from build123d import *

# Parameters (mm, degrees)
SKETCH1_R           = 10
BOSS_EXTRUDE1_DEPTH = 24


with BuildPart() as part:
    # Sketch1 → Boss-Extrude1 (new body)
    with BuildSketch(Plane.XY):
        with BuildLine():
            Line((24.140215409, 6.5), (11.587303396, 53.12))
            ThreePointArc((11.587303396, 53.12), (0, 62), (-11.587303396, 53.12))
            Line((-11.587303396, 53.12), (-24.140215409, 6.5))
            ThreePointArc((-24.140215409, 6.5), (-24.936514863, 1.780512988), (-24.81883517, -3.004233816))
            ThreePointArc((-24.81883517, -3.004233816), (-30.762049538, -19.776348187), (-47.717387131, -25.174694658))
            ThreePointArc((-47.717387131, -25.174694658), (-61.385060233, -49.766289136), (-35, -40))
            ThreePointArc((-35, -40), (-25.668051324, -25.370335536), (-8.412024081, -23.542256707))
            ThreePointArc((-8.412024081, -23.542256707), (0, -25), (8.412024081, -23.542256707))
            ThreePointArc((8.412024081, -23.542256707), (25.668051324, -25.370335536), (35, -40))
            ThreePointArc((35, -40), (61.385060233, -49.766289136), (47.717387131, -25.174694658))
            ThreePointArc((47.717387131, -25.174694658), (30.762049538, -19.776348187), (24.81883517, -3.004233816))
            ThreePointArc((24.81883517, -3.004233816), (24.936514863, 1.780512988), (24.140215409, 6.5))
        make_face()
        with Locations((50, -40)):
            Circle(SKETCH1_R, mode=Mode.SUBTRACT)
        with Locations(Location((-50, -40, 0), (0, 0, 180))):
            Circle(SKETCH1_R, mode=Mode.SUBTRACT)
        with BuildLine():
            Line((4.769696007, 51.5), (19.078784028, 6))
            ThreePointArc((19.078784028, 6), (0, -20), (-19.078784028, 6))
            Line((-19.078784028, 6), (-4.769696007, 51.5))
            ThreePointArc((-4.769696007, 51.5), (0, 55), (4.769696007, 51.5))
        make_face(mode=Mode.SUBTRACT)
    extrude(amount=BOSS_EXTRUDE1_DEPTH)


solid = part.part
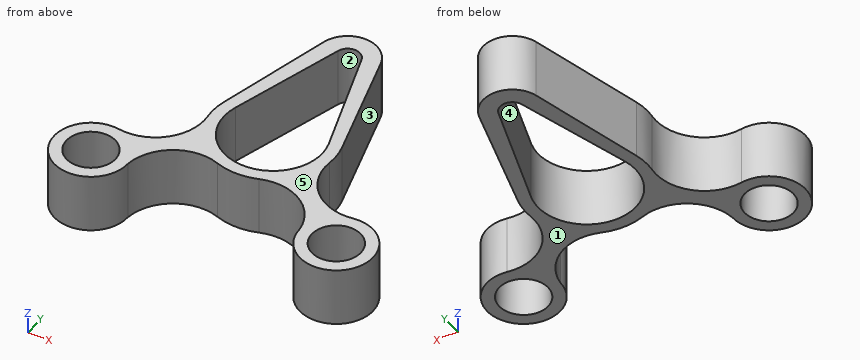
Can you work these out from the model? Positions are in its coordinate system, mm. Face numbers are marked on the shaded views. A direction names the side the tool comes from. Round coordinates to 2 decimals unless told otherwise and drop trailing zeros. Write each loop counter-clockwise with the first axis right and the second up, starting at its lowest first coordinate (ties: lowest second). Pieces come first, ordered by that corner, then holes. Notation, with made-up numbers: (-38, 10.25) -> (21, 10.25) arc R18 ccw to (21, 18.25) -> close; hole circle Ø10 at (-23.75, -3). An arc over 180 degrees is marked (long way). One line per question, with ' | ' between items. Start each with the question number.
1) I'm going to push flat-ended pins straight in: P1, Ø12, axis at y = 19.5, z = 20.5, coming from the +X side; P2, Ø1, axis at y = 25.5, z = 19, coming from the -X side; P3, Ø10, axis at x = 10, y = 46.5, coming from the -Z side; P4, Ø12, axis at x = -50, y = -40, coming from the -Z side. Where does each tip first touch, or does it pass through?
2) Suppose I cut it at A-A on y = 0. Write out the boundary of the cut face in (x, z), then the cut area to 3 significant figures.
3) Suppose I cut it at C-C on z = 19.75. Write out the boundary of the cut face in (x, y), then the cut area to 3 significant figures.
4) I need wall thicknesses on line 1 (Y direction, x = 0, z = 8.75); line 2 (Y direction, x = -50, z = 7.75); line 3 (X direction, y = 0, z = 7). Which ranges of each line are inside material? Lowest first, please. Write a range as [from, to].
5) If we mould it in two halves opening along Y, with no side actions, what happens to the marked faces 1, 2 and 3? For each: released by +Y, released by -Y, zero draft, split by the parting line, or undercut.
6) On a 3-axis mill with a long thin cutter (end or side, diameter ignored), from which of +Z, -Z, +X, -X, +Y, -Y can I reach the whole of each face in a straight line? I mean the marked faces 4 and 5. Say none if no direction works.
7) Suppose I cut it at B-B on x = -50. Write out the boundary of the cut face in (y, z).
Return value:
1) P1: stops at x = 22.26 | P2: stops at x = -19.16 | P3: stops at z = 0 | P4: passes through
2) outline: (-25, 0) -> (-20, 0) -> (-20, 24) -> (-25, 24) -> close; (20, 0) -> (25, 0) -> (25, 24) -> (20, 24) -> close | area: 240 mm2
3) outline: (-47.72, -25.17) arc R15 ccw (long way) to (-35, -40) arc R20 cw to (-8.41, -23.54) arc R25 ccw to (8.41, -23.54) arc R20 cw to (35, -40) arc R15 ccw (long way) to (47.72, -25.17) arc R20 cw to (24.82, -3) arc R25 ccw to (24.14, 6.5) -> (11.59, 53.12) arc R12 ccw to (-11.59, 53.12) -> (-24.14, 6.5) arc R25 ccw to (-24.82, -3) arc R20 cw to start; hole circle Ø20 at (-50, -40); hole (-19.08, 6) arc R20 ccw (long way) to (19.08, 6) -> (4.77, 51.5) arc R5 ccw to (-4.77, 51.5) -> close; hole circle Ø20 at (50, -40) | area: 2,460 mm2
4) line 1: y = [-25, -20], [55, 62] | line 2: y = [-55, -50], [-30, -25] | line 3: x = [-25, -20], [20, 25]
5) face 1: zero draft | face 2: undercut | face 3: released by +Y
6) face 4: +Z, -Z | face 5: +Z, +X, -X, +Y, -Y
7) outline: (-55, 0) -> (-50, 0) -> (-50, 24) -> (-55, 24) -> close; (-30, 0) -> (-25, 0) -> (-25, 24) -> (-30, 24) -> close
